The model under review builds one solid part; all positions refer to its coordinate system, in mm. Give positions to 0.01 mm unless a question says otherwise; leave off trailing zeros. Write each loop counter-clockwise with the first axis right and the second up, starting at its lowest first coordinate (ties: lowest second). Pieces come first, ordered by that corner, then holes. Notation, with made-up numbers: (-13.5, -27.75) -> (-6.5, -27.75) arc R8 ccw to (-6.5, -16.75) -> close; hole circle Ø11 at (-13, -15). An arc over 180 degrees is marked (long way). Use CSV: the item, a comma, the result in double quotes.
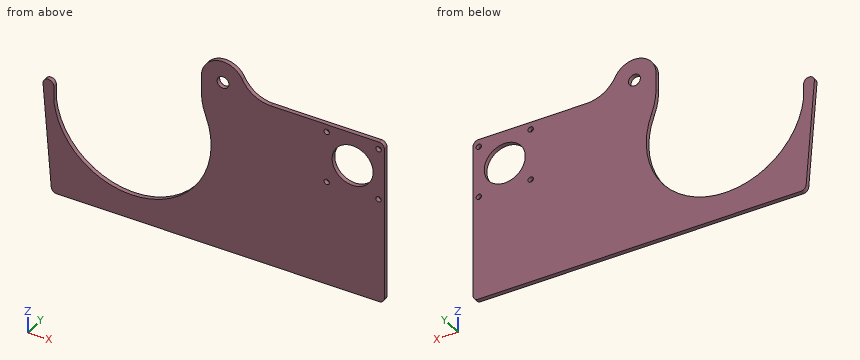
```python
from build123d import *

# Parameters (mm, degrees)
PAD_DEPTH     = 4
SKETCH002_R   = 19
SKETCH002_R_2 = 2.5
SKETCH002_R_3 = 5.5
POCKET_DEPTH  = 4.001
FILLET001_R   = 5


with BuildPart() as part:
    # Sketch001 → Pad (new body)
    with BuildSketch(Plane.XZ):
        with BuildLine():
            Line((-82.604054, 6), (-74.604054, -96))
            Line((-74.604054, -96), (233.395946, -96))
            Line((233.395946, -96), (233.395946, 57))
            Line((233.395946, 57), (128.395946, 57))
            ThreePointArc((101.758378, 73.2), (112.807488, 61.367989), (128.395946, 57))
            ThreePointArc((101.758378, 73.2), (79.265423, 83.431515), (64, 64))
            Line((64, 64), (64, 48.093659))
            ThreePointArc((64, 48.093659), (65.023772, 37.057151), (68.06015, 26.397271))
            ThreePointArc((-72.604054, -7.592846), (17.146247, -70.957778), (68.06015, 26.397271))
            Line((-72.604054, 6), (-72.604054, -7.592846))
            ThreePointArc((-72.604054, 6), (-77.604054, 11), (-82.604054, 6))
        make_face()
    extrude(amount=PAD_DEPTH)

    # Sketch002 → Pocket (cut, through all)
    with BuildSketch(Plane.XZ.offset(4)):
        with Locations((204, 26)):
            Circle(SKETCH002_R)
        with Locations((180, 50)):
            Circle(SKETCH002_R_2)
        with Locations((228, 50)):
            Circle(SKETCH002_R_2)
        with Locations((228, 2)):
            Circle(SKETCH002_R_2)
        with Locations((180, 2)):
            Circle(SKETCH002_R_2)
        with Locations((84, 64)):
            Circle(SKETCH002_R_3)
    extrude(amount=-POCKET_DEPTH, mode=Mode.SUBTRACT)

    # Fillet001
    fillet001_edges = [part.edges().sort_by_distance(p)[0] for p in [
        (233.395946, -2, 57),
        (233.395946, -2, -96),
        (-74.604054, -2, -96),
    ]]
    fillet(fillet001_edges, radius=FILLET001_R)


with BuildPart() as part_1:
    # Body004 placement: moved
    add(part.part.moved(Location((0, 9, 0))))


solid = part_1.part
```
Q1. Consider section C-C (z = -26). Write out the cut boundary in (x, y), then the cut area to 3 significant figures.
Derived:
outline,"(-80.09, 5) -> (-68.21, 5) -> (-68.21, 9) -> (-80.09, 9) -> close; (68.21, 5) -> (233.4, 5) -> (233.4, 9) -> (68.21, 9) -> close"
area,"708 mm2"
Q2. Consider section B-B (y = 8.2). Write out the cut boundary in (x, z).
Derived:
outline,"(-82.6, 6) -> (-74.97, -91.39) arc R5 ccw to (-69.98, -96) -> (228.4, -96) arc R5 ccw to (233.4, -91) -> (233.4, 52) arc R5 ccw to (228.4, 57) -> (128.4, 57) arc R30 cw to (101.76, 73.2) arc R20 ccw to (64, 64) -> (64, 48.09) arc R60 ccw to (68.06, 26.4) arc R73 cw (long way) to (-72.6, -7.59) -> (-72.6, 6) arc R5 ccw to start; hole circle Ø11 at (84, 64); hole circle Ø5 at (180, 2); hole circle Ø5 at (180, 50); hole circle Ø38 at (204, 26); hole circle Ø5 at (228, 2); hole circle Ø5 at (228, 50)"
Q3. To check wall thickness, follow probe 1 along Z at (x, y) = (228, 6.4); probe 2 along X at (y, z) = (8.05, 0); probe 3 along Z at (x, y) = (84, 6.2). State the ranges of each line that lie inside material, in increasing order.
Derived:
probe 1,"z = -96 to -0.5, 4.5 to 47.5, 52.5 to 57"
probe 2,"x = -82.13 to -72.6, 73 to 178.5, 181.5 to 226.5, 229.5 to 233.4"
probe 3,"z = -96 to 58.5, 69.5 to 84"
Q4. Consider section D-D (x = 0). Write out the cut boundary in (y, z).
Derived:
outline,"(5, -96) -> (9, -96) -> (9, -73) -> (5, -73) -> close"
Q5. Consider section A-A (x = 204). Write out the cut boundary in (y, z).
Derived:
outline,"(5, -96) -> (9, -96) -> (9, 7) -> (5, 7) -> close; (5, 45) -> (9, 45) -> (9, 57) -> (5, 57) -> close"
